from build123d import *

# Parameters (mm, degrees)
SKETCH13_R          = 4.7625
BOSS_EXTRUDE1_DEPTH = 6.35
FILLET1_START       = -1
FILLET1_DEPTH       = 8
FILLET2_R           = 25.4


with BuildPart() as part:
    # Sketch13 → Boss-Extrude1 (new body)
    with BuildSketch(Plane(origin=(0, 0, 0), x_dir=(1, 0, 0), z_dir=(0, 1, 0))):
        with BuildLine():
            Line((12.169749373, 58.041291034), (21.253749792, 27.59863924))
            Line((21.253749792, 27.59863924), (13.899399026, -3.307470782))
            ThreePointArc((13.899399026, -3.307470782), (0, -14.2875), (-13.899399026, -3.307470782))
            Line((-13.899399026, -3.307470782), (-21.253749792, 27.59863924))
            Line((-21.253749792, 27.59863924), (-12.169749373, 58.041291034))
            ThreePointArc((-12.169749373, 58.041291034), (0, 41.709872551), (12.169749373, 58.041291034))
        make_face()
        with Locations(Location((0, 0, 0), (0, 0, 270))):
            Circle(SKETCH13_R, mode=Mode.SUBTRACT)
    extrude(amount=BOSS_EXTRUDE1_DEPTH)

    # Fillet1: read off the stored shape, not the designer's step
    # Fillet1 outline → Fillet1 (cut)
    with BuildSketch(Plane(origin=(0, 0, 0), x_dir=(1, 0, 0), z_dir=(0, 1, 0)).offset(FILLET1_START)):
        with BuildLine():
            ThreePointArc((12.169749373, 58.041291034), (12.591930806, 52.756609539), (10.819865776, 47.760022584))
            ThreePointArc((10.819865776, 47.760022584), (13.314491534, 48.948438752), (15.417788806, 47.156336287))
            Line((15.417788806, 47.156336287), (12.169749373, 58.041291034))
        make_face()
        with BuildLine():
            ThreePointArc((-15.417788806, 47.156336287), (-13.314491534, 48.948438752), (-10.819865776, 47.760022584))
            ThreePointArc((-10.819865776, 47.760022584), (-12.591930806, 52.756609539), (-12.169749373, 58.041291034))
            Line((-12.169749373, 58.041291034), (-15.417788806, 47.156336287))
        make_face()
    extrude(amount=FILLET1_DEPTH, mode=Mode.SUBTRACT)

    # Fillet2
    fillet2_edges = [part.edges().sort_by_distance(p)[0] for p in [
        (21.253749792, 3.175, -27.59863924),
        (-21.253749792, 3.175, -27.59863924),
    ]]
    fillet(fillet2_edges, radius=FILLET2_R)


solid = part.part
Design review of the part built by this model. Coordinates are the model's own, in mm. Give positions to 0.01 mm unless a question says otherwise; leave off trailing zeros. Loops run counter-clockwise (first coordinate to the right, second up) from the corner with the lowest first, then second, coordinate; pieces in that order, holes last. Notation, with made-up numbers: M 58.25,25.25 L 111.25,25.25 A14 ccw 111.25,51.25 Z; hole C 46,24 d5. An arc over 180 degrees is marked long. One line per question, with ' | ' between items. Start each with the question number.
1. Add section C-C (z = -1). Write out the cut boundary in (x, y).
2. To check wall thickness, follow L1, parallel to X at y = 1.75, z = -1.5; L2, parallel to X at y = 3.5, z = 2; L3, parallel to Z at x = -3.5, y = 3.75. State the ranges of each line that lie inside material, in increasing order.
3. Add section B-B (x = 2). Write out the cut boundary in (y, z), plus the area to 3 significant figures.
4. Insertion check: P1, Ø3, axis at y = 2.5, z = -5, coming from the -X side; P2, Ø12, axis at x = -0.5, z = -23.5, coming from the -Y side; P3, Ø7.5, axis at x = 0, z = 0, coming from the +Y side; P4, Ø3, axis at y = 2, z = -4.5, coming from the -X side. Each pin has a flat end and moves straight along its axis. Give the tip position at first contact, or say it passes through.
5. Add section D-D (z = -19). Write out the cut boundary in (x, y), plus the area to 3 significant figures.
6. Add section A-A (y = 4.5). Write out the cut boundary in (x, z) (1 decimal).
Worked out:
1) outline: M -14.92,0 L -4.66,0 L -4.66,6.35 L -14.92,6.35 Z; M 4.66,0 L 14.92,0 L 14.92,6.35 L 4.66,6.35 Z
2) L1: x = -15.04 to -4.52, 4.52 to 15.04 | L2: x = -14.21 to -4.32, 4.32 to 14.21 | L3: z = -42.2 to -3.23, 3.23 to 13.85
3) outline: M 0,-41.87 L 6.35,-41.87 L 6.35,-4.32 L 0,-4.32 Z; M 0,4.32 L 6.35,4.32 L 6.35,14.15 L 0,14.15 Z | area: 301 mm²
4) P1: stops at x = -16.23 | P2: stops at y = 0 | P3: passes through | P4: stops at x = -16.11
5) outline: M -19.21,0 L 19.21,0 L 19.21,6.35 L -19.21,6.35 Z | area: 244 mm²
6) outline: M -19.7,-21 A25.4 ccw -19.3,-34.1 L -15.4,-47.2 A2.5 ccw -10.8,-47.8 A12.7 cw 10.8,-47.8 A2.5 ccw 15.4,-47.2 L 19.3,-34.1 A25.4 ccw 19.7,-21 L 13.9,3.3 A14.3 ccw -13.9,3.3 Z; hole C 0,0 d9.5
